Build history of the part. All positions in model axes, mm. A direction names the side the tool comes from. Give positions to 0.01 mm unless a question says otherwise; leave off trailing zeros. Write each loop counter-clockwise with the first axis right and the second up, starting at its lowest first coordinate (ties: lowest second). Pieces come first, ordered by that corner, then holes.
from build123d import *


with BuildPart() as f1:
    # F0 (on Front) → F1 (revolve)
    with BuildSketch(Plane.XZ):
        with BuildLine():
            Line((-8.854447, -18.343976), (0, -18.343976))
            Line((0, -18.343976), (0, -17.835976))
            Line((0, -17.835976), (-8.367852, -17.835976))
            Line((-8.367852, -17.835976), (-10.812766, 38.940323))
            ThreePointArc((-10.812766, 38.940323), (-9.989486, 43.872899), (-7.239652, 48.049801))
            ThreePointArc((-7.239652, 48.049801), (-4.731806, 52.564304), (-5.041906, 57.719287))
            Line((-5.041906, 57.719287), (-5.583482, 57.719287))
            ThreePointArc((-5.583482, 57.719287), (-5.207415, 52.765972), (-7.596975, 48.410888))
            ThreePointArc((-7.596975, 48.410888), (-10.462407, 44.058398), (-11.320296, 38.918467))
            Line((-11.320296, 38.918467), (-8.854447, -18.343976))
        make_face()
    revolve(axis=Axis((0, 0, -19.859783), (0, 0, 1)))


solid = f1.part
1. Drop flat-ended pins along their axis: pin 1 (5 mm diameter, centred on x = 0, z = 17, fed in from +Y); pin 2 (6 mm diameter, centred on x = 2, z = -9.5, fed in from -Y); pin 3 (4 mm diameter, centred on x = 6.5, y = 2, fed in from +Z); pin 4 (1 mm diameter, centred on x = -4, z = 37.5, fed in from +Y). Give the stop position or say it passes through.
2. Saw through at A-A on z = 1. Give the cut face in (x, y).
3. Drill centre lines: line 1 along X through (y, z) = (5.25, -1); line 2 along Z through (x, y) = (1.75, 3.5); line 3 along X through (y, z) = (-9, 25.5). Where is each one in solid material? Low to high.
4. Mould opens along Z. For faces 3 (the face through (0, 0, -18.344)), 4 (the face through (-9.164, -2.886, 10.95)) say: pulls with the +Z half, pulls with the -Z half, needs draft (parallel to the pull), parting line crosses it, or undercut.
5. 3-axis set-ups, long thin cutter, end or side, ignore diameter. For faces 1 (the face through (-9.605, -3.025, 9.886)), 2 (the face through (0, 0, -17.836)): which of +Z, -Z, +X, -X, +Y, -Y reach the whole face in a straight line?
Outcome:
1. pin 1: stops at y = 10.48
1. pin 2: stops at y = -9.34
1. pin 3: stops at z = 57.72
1. pin 4: stops at y = 10.7
2. outline: circle Ø19.37 at (0, 0); hole circle Ø18.36 at (0, 0)
3. line 1: x = -8.04 to -7.42, 7.42 to 8.04
3. line 2: z = -18.34 to -17.84
3. line 3: x = -5.87 to -4.87, 4.87 to 5.87
4. face 3: pulls with the -Z half
4. face 4: undercut
5. face 1: -Z
5. face 2: none
